Geometry check sheet. Reference: the model listing, model coordinates, mm. Face numbers are marked on the shaded views. A direction names the side the tool comes from. Coordinates: 2 decimals unless noted, no trailing zeros. Order: outer loops, then holes, each group sorted by start corner. A loop starts at its lowest first (then second) coordinate and runs counter-clockwise, first axis right, second up. Notation, with made-up numbers: (13.5, -21.5) -> (39.5, -21.5) arc R9 cw to (39.5, -10.5) -> close; hole circle Ø6 at (-29, -36). An arc over 180 degrees is marked (long way). Answer as CSV lines item,"result". Start each with the question number.
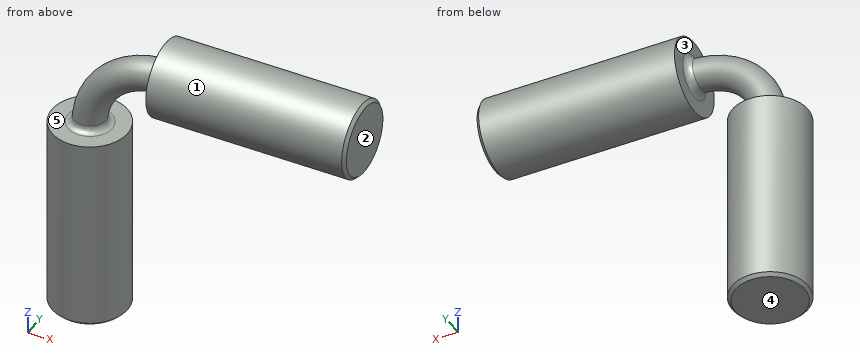
from build123d import *

# Parameters (mm, degrees)
SWEEP2_PROFILE_R     = 2.5
SKETCH49_R           = 6
BOSS_EXTRUDE9_DEPTH  = 31.5
SKETCH54_R           = 6
BOSS_EXTRUDE10_DEPTH = 31.5
FILLET32_R           = 1
FILLET33_R           = 1
CHAMFER1_SIZE        = 0.5
CHAMFER2_SIZE        = 0.5


with BuildPart() as part:
    # Sweep2: sweep along a path in Sketch1
    with BuildLine(Plane(origin=(0, 0, 0), x_dir=(1, 0, 0), z_dir=(0, 1, 0))) as sweep2_path:
        Line((0, 31.5), (0, 0))
        ThreePointArc((0, 0), (3.514718626, -8.485281374), (12, -12))
        Line((12, -12), (43.5, -12))
    # Sweep2 profile (on start of the path) → Sweep2 (sweep)
    with BuildSketch(Plane.XY.offset(-31.5)):
        Circle(SWEEP2_PROFILE_R)
    sweep(path=sweep2_path.line)

    # Sketch49 → Boss-Extrude9 (add)
    with BuildSketch(Plane(origin=(43.5, 0, 0), x_dir=(0, 0, -1), z_dir=(1, 0, 0))):
        with Locations((-12, 0)):
            Circle(SKETCH49_R)
    extrude(amount=-BOSS_EXTRUDE9_DEPTH)

    # Sketch54 → Boss-Extrude10 (add)
    with BuildSketch(Plane(origin=(0, 0, -31.5), x_dir=(-1, 0, 0), z_dir=(0, 0, -1))):
        Circle(SKETCH54_R)
    extrude(amount=-BOSS_EXTRUDE10_DEPTH)

    # Fillet32
    fillet32_edges = [part.edges().sort_by_distance(p)[0] for p in [
        (12, 0, 14.5),
    ]]
    fillet(fillet32_edges, radius=FILLET32_R)

    # Fillet33
    fillet33_edges = [part.edges().sort_by_distance(p)[0] for p in [
        (-2.5, 0, 0),
    ]]
    fillet(fillet33_edges, radius=FILLET33_R)

    # Chamfer1
    chamfer1_edges = [part.edges().sort_by_distance(p)[0] for p in [
        (43.5, 0, 18),
    ]]
    chamfer(chamfer1_edges, length=CHAMFER1_SIZE)

    # Chamfer2
    chamfer2_edges = [part.edges().sort_by_distance(p)[0] for p in [
        (6, 0, -31.5),
    ]]
    chamfer(chamfer2_edges, length=CHAMFER2_SIZE)


solid = part.part
Q1. Sectioned sample at A-A, the plane x = 14.5. Record the cut outline in (y, z).
Q2. Access from +Z, -Z, +X, -X, +Y, -Y to the whole of each face (thin tool, end or side, straight path). Record for the marked faces 4 and 5.
Q3. Release check for a two-part mould opening along X. For the marked faces 1, 2 and 3 record: released by +X, released by -X, zero draft, split by the parting line, or undercut.
Q4. Go/stop test with flat-tipped pins: pin 1 Ø4 at (x, y) = (35.5, -4) entering from -Z; pin 2 Ø1 at (y, z) = (1, -8.5) entering from +X; pin 3 Ø1 at (x, y) = (31.5, -4) entering from +Z. Record where each tip stops, or that it passes through.
Q5. Sectioned sample at B-B, the plane z = -8. Record the cut outline in (x, y).
Q6. Thickness scan on L1, parallel to Y at x = 14.5, z = 6.5; L2, parallel to Z at x = 16, y = 0.25; L3, parallel to X at y = -5, z = -27.5. Record the ranges inside material, lowest first.
Geometry results:
1,outline,"circle Ø12 at (0, 12)"
2,face 4,"-Z, +X, -X, +Y, -Y"
2,face 5,"none"
3,face 1,"zero draft"
3,face 2,"released by +X"
3,face 3,"undercut"
4,pin 1,"stops at z = 6.34"
4,pin 2,"stops at x = 5.98"
4,pin 3,"stops at z = 16.87"
5,outline,"circle Ø12 at (0, 0)"
6,L1,"y = -2.4 to 2.4"
6,L2,"z = 6.01 to 17.99"
6,L3,"x = -3.32 to 3.32"
